Here's how the part is built. I have some questions about the finished solid (model axes, mm). A direction names the side the tool comes from. Round coordinates to 2 decimals unless told otherwise and drop trailing zeros. Order: outer loops, then holes, each group sorted by start corner. A loop starts at its lowest first (then second) coordinate and runs counter-clockwise, first axis right, second up.
Autodesk Inventor part; units mm, degrees
ref_plane "YZ Plane" through (0, 0, 0) normal (1, 0, 0) x (0, 1, 0)
ref_plane "XZ Plane" through (0, 0, 0) normal (0, 1, 0) x (-1, 0, 0)
ref_plane "XY Plane" through (0, 0, 0) normal (0, 0, 1) x (1, 0, 0)
sketch "Sketch1" plane through (0, 0, 0) normal (0, 0, 1) x (1, 0, 0)
  line L0 (-63.3984, -65.0875) -> (63.3984, -65.0875)
  line L1 (63.3984, -65.0875) -> (63.3984, 65.0875)
  line L2 (63.3984, 65.0875) -> (-63.3984, 65.0875)
  line L3 (-63.3984, 65.0875) -> (-63.3984, -65.0875)
  line L4 (-63.3984, -65.0875) -> (63.3984, 65.0875) construction
  line L5 (63.3984, -65.0875) -> (-63.3984, 65.0875) construction
  point P0 (0, 0)
  dimension "d0" = 126.7968
  dimension "d1" = 130.175
extrude "Extrusion1" add sketch "Sketch1" along normal blind 9.525
sketch "Sketch2" plane through (0, 0, 9.525) normal (0, 0, 1) x (1, 0, 0)
  circle A0 centre (0, 0) radius 50.8508
  dimension "d4" = 101.7016
extrude "Extrusion2" cut sketch "Sketch2" against normal blind 6.35
sketch "Sketch3" plane through (0, 0, 3.175) normal (0, 0, 1) x (1, 0, 0)
  circle A0 centre (0, 0) radius 47.625
  dimension "d7" = 95.25
extrude "Extrusion3" cut sketch "Sketch3" along normal through all both and the other way through all
equation "\"d0\" = width - 2 * alignmentGrooveClearance"
equation "\"d1\" = height + 2 * alignmentGrooveDepth"
equation "\"d2\" = lensMountThickness"
equation "\"d4\" = lensDiameter + alignmentGrooveClearance"
equation "\"d5\" = lensInsetDepth"
equation "\"d7\" = lensDiameter - lensInsetDepth"
equation "\"d8\" = lensInsetDepth"
equation "\"caseThickness\" = 6.35"
equation "\"alignmentGrooveDepth\" = 1.5875"
equation "\"alignmentGrooveClearance\" = 0.1016"
equation "\"aerogelHolderDepth\" = 38.24501"
equation "\"height\" = 127"
equation "\"width\" = 127"
equation "\"depth\" = 247.57228"
equation "\"mirrorAngle\" = 2.5deg"
equation "\"mirrorThickness\" = 3.175"
equation "\"fresnelThickness\" = 0.254"
equation "\"focalLength\" = 185.82488"
equation "\"ior\" = 1.49"
equation "\"centerThickness\" = 1.27"
equation "\"fresnelAngle\" = 90deg"
equation "\"fresnelEffectiveDiameter\" = 152.4"
equation "\"fresnelGrooveWidth\" = 9.525"
equation "\"frontPanelThickness\" = 1.5875"
equation "\"lensMountThickness\" = 9.525"
equation "\"lensInsetDepth\" = 6.35"
equation "\"lensDiameter\" = 101.6"
equation "\"lensCenterThickness\" = 16.99999"
properties part number "sphericalLensHolder" material "ABS Plastic"
1. I need wall thicknesses on probe 1 along Y at (x, z) = (-1.5, 4); probe 2 along Y at (x, z) = (0, 2.2) (1 decimal); probe 3 along X at (y, z) = (9.5, 5.25). Which ranges of each line are inside material? Lowest first, please.
Evaluation:
probe 1: y = -65.09 to -50.83, 50.83 to 65.09
probe 2: y = -65.1 to -47.6, 47.6 to 65.1
probe 3: x = -63.4 to -49.96, 49.96 to 63.4
2. If we section it at C-C, the plane z = 7: Write out the boundary of the cut face in (x, y).
Evaluation:
outline: (-63.4, -65.09) - (63.4, -65.09) - (63.4, 65.09) - (-63.4, 65.09) - close; hole circle Ø101.7 at (0, 0)
3. On a 3-axis mill with a long thin cutter (end or side, diameter ignored), from which of +Z, -Z, +X, -X, +Y, -Y can I reach the whole of each face in a straight line? I mean faces 1 (the cylindrical face through (27.3, 42.9, 6.4)), 2 (the flat face through (1, 65.088, 5)). Say none if no direction works.
Evaluation:
face 1: +Z
face 2: +Z, -Z, +X, -X, +Y
4. If we section it at A-A, the plane x = 0: Write out the boundary of the cut face in (y, z) (1 decimal).
Evaluation:
outline: (-65.1, 0) - (-47.6, 0) - (-47.6, 3.2) - (-50.9, 3.2) - (-50.9, 9.5) - (-65.1, 9.5) - close; (47.6, 0) - (65.1, 0) - (65.1, 9.5) - (50.9, 9.5) - (50.9, 3.2) - (47.6, 3.2) - close
5. I'm going to push a flat-ended pin straight in: P1, Ø4, axis at x = 45.5, y = -18, coming from the -Z side. Where does the tip first touch, or does it pass through?
Evaluation:
P1: stops at z = 0
6. If we mould it in two halves opening along Y, with no side actions, what happens to faces 3 (the flat face through (-1, -65.088, 5)), 4 (the flat face through (14.83, 45.44, 3.175)), 5 (the flat face through (-63.398, 1, 5))? For each: released by +Y, released by -Y, zero draft, split by the parting line, or undercut.
Evaluation:
face 3: released by -Y
face 4: undercut
face 5: zero draft
7. If we section it at B-B, the plane y = 0: Write out the boundary of the cut face in (x, z) (3 decimals).
Evaluation:
outline: (-63.398, 0) - (-47.625, 0) - (-47.625, 3.175) - (-50.851, 3.175) - (-50.851, 9.525) - (-63.398, 9.525) - close; (47.625, 0) - (63.398, 0) - (63.398, 9.525) - (50.851, 9.525) - (50.851, 3.175) - (47.625, 3.175) - close
